The model under review builds one solid part; all positions refer to its coordinate system, in mm. A direction names the side the tool comes from. Round coordinates to 2 decimals unless told otherwise and drop trailing zeros. Order: outer loops, then holes, each group sorted by start corner. A loop starts at its lowest first (then second) coordinate and runs counter-clockwise, first axis right, second up.
1) Clearance check with flat-ended pins moving along their axes: P1, Ø2, axis at x = 29.5, y = 29.5, coming from the +Z side; P2, Ø2, axis at y = 23, z = -64.5, coming from the +X side; P3, Ø1.3, axis at x = 96.5, z = -78.5, coming from the +Y side. State where each tip first meets the part, or that it passes through.
2) To check wall thickness, follow L1, parallel to X at y = 33.3, z = -3; L2, parallel to X at y = 22, z = -4.5; L3, parallel to Z at x = 37, y = 14. State the ranges of each line that lie inside material, in increasing order.
3) Consider section A-A (y = 22.5). Give the boundary of the cut face in (x, z).
4) Machinability: for faces 4 (the face through (49, 17, -79)), 5 (the face through (49, 17, -3)), 6 (the face through (3, 31, -79)), which of the approach directions +Z, -Z, +X, -X, +Y, -Y give a long, thin tool a straight path to every point of the face, cutting with its end or side? Answer none if there is none.
5) Consider section B-B (x = 63). Give the boundary of the cut face in (y, z), then the cut area to 3 significant figures.
6) Mouldability with a two-part tool opening along Y and no side actions: class faces 1 (the face through (49, 32, -1)), 2 (the face through (0.804, 32.521, -3.488)), 3 (the face through (49, 34, -42)) as pulls with the +Y half, pulls with the -Y half, needs draft (parallel to the pull), parting line crosses it, or undercut.
from build123d import *

# Parameters (mm, degrees)
SKETCH1_W                = 100
SKETCH1_H                = 82
BOSS_EXTRUDE1_DEPTH      = 34
SKETCH2_W                = 96
SKETCH2_H                = 30
CUT_EXTRUDE1_DEPTH       = 3
CHAMFER1_SIZE            = 5
CHAMFER1_OF_MIRROR4_SIZE = 5
SKETCH3_R                = 2.25
CUT_EXTRUDE2_DEPTH       = 3
SKETCH4_W                = 35
SKETCH4_H                = 12
BOSS_EXTRUDE2_DEPTH      = 1


with BuildPart() as part:
    # Sketch1 → Boss-Extrude1 (new body)
    with BuildSketch(Plane(origin=(0, 0, 0), x_dir=(1, 0, 0), z_dir=(0, 1, 0))):
        with Locations((50, 41)):
            Rectangle(SKETCH1_W, SKETCH1_H)
    extrude(amount=BOSS_EXTRUDE1_DEPTH)

    # Sketch2 → Cut-Extrude1 (cut)
    with BuildSketch(Plane.XY):
        with Locations((50, 17)):
            Rectangle(SKETCH2_W, SKETCH2_H)
    cut_extrude1 = extrude(amount=-CUT_EXTRUDE1_DEPTH, mode=Mode.SUBTRACT)

    # Chamfer1
    chamfer1_edges = [part.edges().sort_by_distance(p)[0] for p in [
        (2, 32, -1.5),
        (98, 32, -1.5),
    ]]
    chamfer(chamfer1_edges, length=CHAMFER1_SIZE)

    # Mirror4: Cut-Extrude1 across plane
    add(cut_extrude1.mirror(Plane.XY.offset(-41)), mode=Mode.SUBTRACT)

    # Chamfer1 of Mirror4
    chamfer1_of_mirror4_edges = [part.edges().sort_by_distance(p)[0] for p in [
        (2, 32, -80.5),
        (98, 32, -80.5),
    ]]
    chamfer(chamfer1_of_mirror4_edges, length=CHAMFER1_OF_MIRROR4_SIZE)

    # Sketch3 → Cut-Extrude2 (cut)
    with BuildSketch(Plane(origin=(0, 34, 0), x_dir=(1, 0, 0), z_dir=(0, 1, 0))):
        with Locations(Location((3, 79, 0), (0, 0, 270))):
            Circle(SKETCH3_R)
        with Locations(Location((3, 3, 0), (0, 0, 270))):
            Circle(SKETCH3_R)
        with Locations(Location((97, 3, 0), (0, 0, 270))):
            Circle(SKETCH3_R)
        with Locations(Location((97, 79, 0), (0, 0, 270))):
            Circle(SKETCH3_R)
    extrude(amount=-CUT_EXTRUDE2_DEPTH, mode=Mode.SUBTRACT)

    # Sketch4 → Boss-Extrude2 (add)
    with BuildSketch(Plane(origin=(100, 0, 0), x_dir=(0, 0, -1), z_dir=(1, 0, 0))):
        with Locations((41, 26.5)):
            Rectangle(SKETCH4_W, SKETCH4_H)
    extrude(amount=BOSS_EXTRUDE2_DEPTH)


solid = part.part
Answer below:
1. P1: stops at z = -3
1. P2: stops at x = 100
1. P3: stops at y = 31
2. L1: x = 0 to 0.75, 5.25 to 94.75, 99.25 to 100
2. L2: x = 0 to 100
2. L3: z = -79 to -3
3. outline: (0, -82) - (2, -82) - (2, -79) - (98, -79) - (98, -82) - (100, -82) - (100, -58.5) - (101, -58.5) - (101, -23.5) - (100, -23.5) - (100, 0) - (98, 0) - (98, -3) - (2, -3) - (2, 0) - (0, 0) - close
4. face 4: -Z
4. face 5: +Z
4. face 6: +Y
5. outline: (0, -82) - (2, -82) - (2, -79) - (32, -79) - (32, -82) - (34, -82) - (34, 0) - (32, 0) - (32, -3) - (2, -3) - (2, 0) - (0, 0) - close
5. area: 2,610 mm2
6. face 1: undercut
6. face 2: needs draft
6. face 3: pulls with the +Y half
